Here's how the part is built. I have some questions about the finished solid (model axes, mm). Face numbers are marked on the shaded views. A direction names the side the tool comes from. Coordinates: 2 decimals unless noted, no trailing zeros. Write each loop counter-clockwise with the first axis right and the second up, starting at its lowest first coordinate (ties: lowest second). Pieces come first, ordered by that corner, then holes.
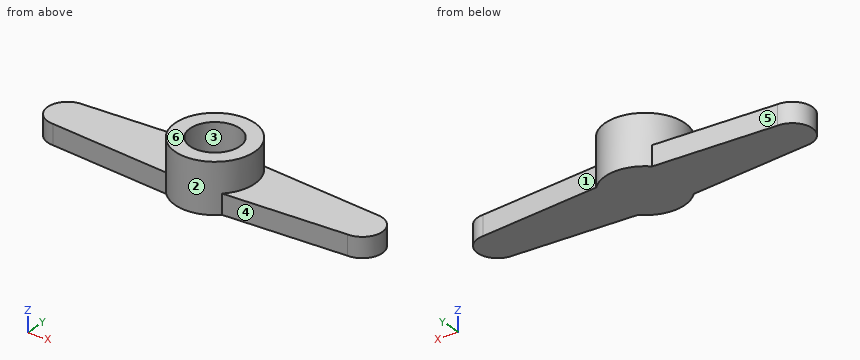
from build123d import *

# Parameters (mm, degrees)
CYLINDER001_R     = 2.5
CYLINDER001_DEPTH = 3
CYLINDER_R        = 4
CYLINDER_DEPTH    = 5
PAD_DEPTH         = 2


with BuildPart() as cylinder001:
    # Cylinder001 → Cylinder001 (new body)
    with BuildSketch(Plane.XY.offset(2)):
        Circle(CYLINDER001_R)
    extrude(amount=CYLINDER001_DEPTH)


with BuildPart() as cut:
    # Cylinder → Cylinder (new body)
    with BuildSketch(Plane.XY):
        Circle(CYLINDER_R)
    extrude(amount=CYLINDER_DEPTH)

    # Cut: cut Cylinder001
    add(cylinder001.part, mode=Mode.SUBTRACT)


with BuildPart() as servo_arm:
    # Sketch → Pad (new body)
    with BuildSketch(Plane.XY):
        with BuildLine():
            Line((-15, 2), (0, 3))
            Line((0, 3), (15, 2))
            ThreePointArc((15, -2), (17, 0), (15, 2))
            Line((15, -2), (0, -3))
            Line((0, -3), (-15, -2))
            ThreePointArc((-15, 2), (-17, 0), (-15, -2))
        make_face()
    extrude(amount=PAD_DEPTH)

    # Fusion: union Cut
    add(cut.part)


solid = servo_arm.part
1. I want a section at C-C (y = 0). List the corners of the cut face in (x, z) for me, then the cut area to 3 significant figures.
2. Thinking about a two-plate mould opening in Y: for the marked faces 3, 4, 5 and 6, which applies, pulls with the +Y half, pulls with the -Y half, needs draft (parallel to the pull), parting line crosses it, or undercut?
3. If I drill on line 1 (Y direction, x = 0, z = 3.9); line 2 (Y direction, x = 7.5, z = 1.8); line 3 (Z direction, x = 13.5, y = -2), over which ranges is the centre line in solid material (lowest first)?
4. I want a section at A-A (x = 0). List the corners of the cut face in (y, z) for me, then the cut area to 3 significant figures.
5. On a 3-axis mill with a long thin cutter (end or side, diameter ignored), from which of +Z, -Z, +X, -X, +Y, -Y can I reach the whole of each face in a straight line? I mean the marked faces 1 and 2. Say none if no direction works.
6. I want a section at D-D (z = 0.65). List the corners of the cut face in (x, y) for me.
7. I want a section at B-B (z = 4.7). List the corners of the cut face in (x, y) for me, then the cut area to 3 significant figures.
8. For pin 1 Ø1 at (x, z) = (4, 1.5) entering from -Y; pin 2 Ø3 at (y, z) = (3, 2) entering from +X; pin 3 Ø1.5 at (x, z) = (2, 4.5) entering from +Y, each with a flat end and sliding along its axis, tell me the tip position at first contact or that it passes through.
Response values:
1. outline: (-17, 0) - (17, 0) - (17, 2) - (4, 2) - (4, 5) - (2.5, 5) - (2.5, 2) - (-2.5, 2) - (-2.5, 5) - (-4, 5) - (-4, 2) - (-17, 2) - close
1. area: 77.0 mm2
2. face 3: undercut
2. face 4: pulls with the -Y half
2. face 5: pulls with the +Y half
2. face 6: needs draft
3. line 1: y = -4 to -2.5, 2.5 to 4
3. line 2: y = -2.5 to 2.5
3. line 3: z = 0 to 2
4. outline: (-4, 0) - (4, 0) - (4, 5) - (2.5, 5) - (2.5, 2) - (-2.5, 2) - (-2.5, 5) - (-4, 5) - close
4. area: 25.0 mm2
5. face 1: +Z, -Z, +X, +Y
5. face 2: +Z
6. outline: (-15, -2) - (-2.85, -2.81) arc R4 ccw to (2.85, -2.81) - (15, -2) arc R2 ccw to (15, 2) - (2.85, 2.81) arc R4 ccw to (-2.85, 2.81) - (-15, 2) arc R2 ccw to start
7. outline: circle Ø8 at (0, 0); hole circle Ø5 at (0, 0)
7. area: 30.6 mm2
8. pin 1: stops at y = -2.77
8. pin 2: stops at x = 16.32
8. pin 3: stops at y = 3.8
